Answer from the drawing. Dimensions are ordinates in mm from the lowest x, y and z of the part. A direction names the side the tool comes from. Give positions to 0.01 mm unless a question says otherwise; leave off trailing zeros. Order: outer loops, then holes, each group sorted by start corner. A loop starts at its lowest first (then second) coordinate and runs counter-clockwise, first axis right, second up.
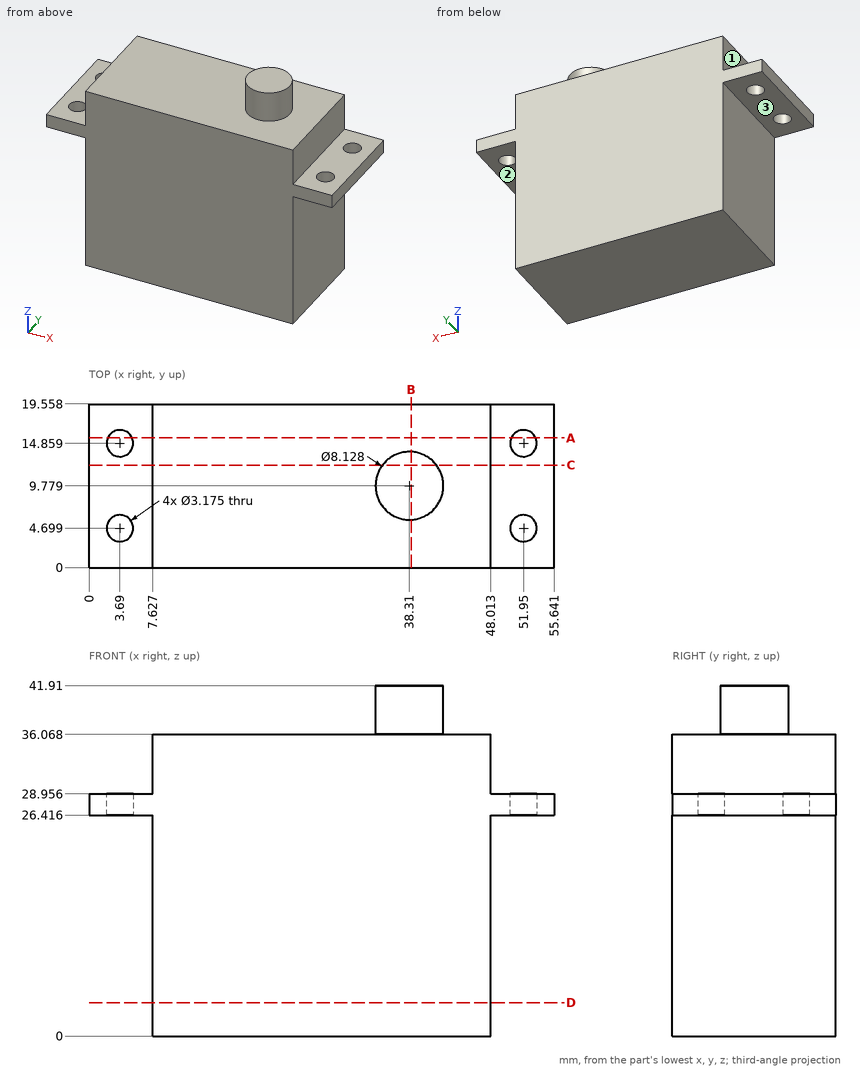
1) The part is cut by section C-C on y = 12.25. Determine the outline of the cut face in (x, z).
Final values:
outline: (0, 26.42) - (7.63, 26.42) - (7.63, 0) - (48.01, 0) - (48.01, 26.42) - (55.64, 26.42) - (55.64, 28.96) - (48.01, 28.96) - (48.01, 36.07) - (41.54, 36.07) - (41.54, 41.91) - (35.08, 41.91) - (35.08, 36.07) - (7.63, 36.07) - (7.63, 28.96) - (0, 28.96) - close
2) Consider L1, parallel to Z at x = 16, y = 14; L2, parallel to Z at x = 50, y = 8.25; L3, parallel to X at y = 10, z = 23. Determine where each line is inside the solid, lowest interval first.
Final values:
L1: z = 0 to 36.07
L2: z = 26.42 to 28.96
L3: x = 7.63 to 48.01
3) The part is cut by section A-A on y = 15.5. Determine the outline of the cut face in (x, z), and give its area (3 significant figures).
Final values:
outline: (0, 26.42) - (2.24, 26.42) - (2.24, 28.96) - (0, 28.96) - close; (5.14, 26.42) - (7.63, 26.42) - (7.63, 0) - (48.01, 0) - (48.01, 26.42) - (50.5, 26.42) - (50.5, 28.96) - (48.01, 28.96) - (48.01, 36.07) - (7.63, 36.07) - (7.63, 28.96) - (5.14, 28.96) - close; (53.4, 26.42) - (55.64, 26.42) - (55.64, 28.96) - (53.4, 28.96) - close
area: 1,480 mm2
4) Given pin 1 (3 mm diameter, centred on x = 16.5, y = 3.5, fed in from +Z); pin 2 (3.5 mm diameter, centred on y = 13.5, z = 32, fed in from +X); pin 3 (3 mm diameter, centred on y = 11, z = 11, fed in from -X), each flat-ended and moving along its own axis, determine where each tip first touches the part or whether it passes through.
Final values:
pin 1: stops at z = 36.07
pin 2: stops at x = 48.01
pin 3: stops at x = 7.63
5) The part is cut by section B-B on x = 38.5. Determine the outline of the cut face in (y, z).
Final values:
outline: (0, 0) - (19.56, 0) - (19.56, 36.07) - (13.84, 36.07) - (13.84, 41.91) - (5.72, 41.91) - (5.72, 36.07) - (0, 36.07) - close
6) A tool of negligible diameter and unlimited length cuts with its end or side. For the marked faces 1, 2 and 3, from which of +Z, -Z, +X, -X, +Y, -Y can it reach the whole face along a straight path? Write none if from no direction.
Final values:
face 1: +Z, -X, +Y, -Y
face 2: -Z, +X, +Y, -Y
face 3: -Z, -X, +Y, -Y
7) The part is cut by section D-D on z = 4. Determine the outline of the cut face in (x, y), and give its area (3 significant figures).
Final values:
outline: (7.63, 0) - (48.01, 0) - (48.01, 19.56) - (7.63, 19.56) - close
area: 790 mm2
